```python
from build123d import *

# Parameters (mm, degrees)
F0_W     = 100
F0_H     = 80
F1_DEPTH = 12
F2_D     = 6.6
F2_DEPTH = 12
F2_TIP   = 1.9828400428
F3_W     = 100
F3_H     = 27.5
F4_DEPTH = 20


with BuildPart() as f1:
    # F0 (on Front) → F1 (new body)
    with BuildSketch(Plane.XZ):
        with Locations((-50, 40)):
            Rectangle(F0_W, F0_H)
    extrude(amount=F1_DEPTH)

    # F2
    with Locations(Plane(origin=(0, 0, 0), x_dir=(1, 0, 0), z_dir=(0, 1, 0))):
        with Locations((-75.5, -40), (-50, -14.5), (-50, -65.5), (-24.5, -40)):
            Hole(F2_D / 2, depth=F2_DEPTH)
            with Locations((0, 0, -(F2_DEPTH + F2_TIP / 2))):  # 118° drill point
                Cone(0, F2_D / 2, F2_TIP, mode=Mode.SUBTRACT)

    # F3 (on face) → F4 (join)
    with BuildSketch(Plane.XZ.offset(12)):
        with Locations((-50, 13.75)):
            Rectangle(F3_W, F3_H)
        with Locations((-50, 66.25)):
            Rectangle(F3_W, F3_H)
    extrude(amount=F4_DEPTH)


solid = f1.part
```
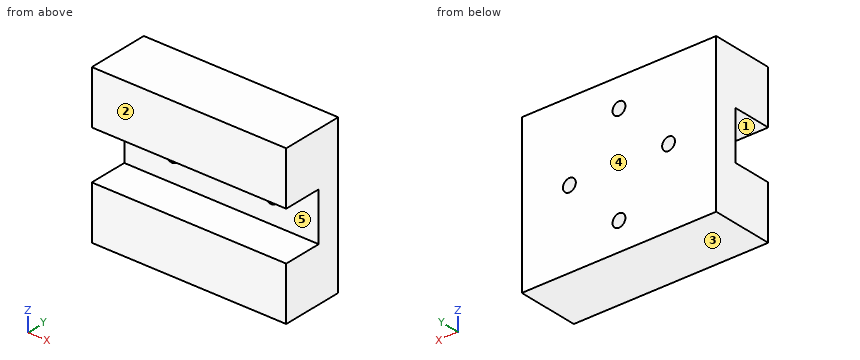
Build history of the part. All positions in model axes, mm. Face numbers are marked on the shaded views. A direction names the side the tool comes from. Give positions to 0.01 mm unless a question says otherwise; leave off trailing zeros. Loops run counter-clockwise (first coordinate to the right, second up) from the corner with the lowest first, then second, coordinate; pieces in that order, holes last.
1) Band-saw the part on B-B on x = -75.5. List the corners of the cut face in (y, z).
Values follow:
outline: (-32, 0) - (0, 0) - (0, 36.7) - (-12, 36.7) - (-12, 27.5) - (-32, 27.5) - close; (-32, 52.5) - (-12, 52.5) - (-12, 43.3) - (0, 43.3) - (0, 80) - (-32, 80) - close
2) Band-saw the part on D-D on z = 65.5. List the corners of the cut face in (x, y), then the cut area to 3 significant figures.
Values follow:
outline: (-100, -32) - (0, -32) - (0, 0) - (-46.7, 0) - (-46.7, -12) - (-53.3, -12) - (-53.3, 0) - (-100, 0) - close
area: 3,120 mm2
3) Two-plate mould, pull along Z, no slides. Class the marked faces 3, 4 and 5: released by +Z, released by -Z, zero draft, split by the parting line, or undercut.
Values follow:
face 3: released by -Z
face 4: zero draft
face 5: undercut
4) Probe line 1 along Z through (x, y) = (-87.5, -19.5); line 2 along X through (y, z) = (-6.75, 14.5); line 3 along Z through (x, y) = (-24.5, -3.5). List the from-to ranges inside material, lowest first.
Values follow:
line 1: z = 0 to 27.5, 52.5 to 80
line 2: x = -100 to -53.3, -46.7 to 0
line 3: z = 0 to 36.7, 43.3 to 80
5) Drop flat-ended pins along their axis: P1, Ø7.5, axis at x = -24.5, z = 40, coming from the -Y side; P2, Ø2, axis at x = -50.5, z = 66.5, coming from the +Y side. Give the stop position or say it passes through.
Values follow:
P1: stops at y = -12
P2: stops at y = -12
6) Band-saw the part on A-A on z = 40. List the corners of the cut face in (x, y).
Values follow:
outline: (-100, -12) - (-78.8, -12) - (-78.8, 0) - (-100, 0) - close; (-72.2, -12) - (-27.8, -12) - (-27.8, 0) - (-72.2, 0) - close; (-21.2, -12) - (0, -12) - (0, 0) - (-21.2, 0) - close
7) Band-saw the part on C-C on y = -17. List the corners of the cut face in (x, z).
Values follow:
outline: (-100, 0) - (0, 0) - (0, 27.5) - (-100, 27.5) - close; (-100, 52.5) - (0, 52.5) - (0, 80) - (-100, 80) - close
8) 3-axis set-ups, long thin cutter, end or side, ignore diameter. For the marked faces 1 and 2: which of +Z, -Z, +X, -X, +Y, -Y reach the whole face in a straight line?
Values follow:
face 1: +X, -X, -Y
face 2: +Z, -Z, +X, -X, -Y
